Could you check a few things on this model? Use its own coordinates, in mm. Face numbers are marked on the shaded views. A direction names the side the tool comes from. Give positions to 0.01 mm unless a question says otherwise; leave off trailing zeros. Loops run counter-clockwise (first coordinate to the right, second up) from the corner with the lowest first, then second, coordinate; pieces in that order, holes last. Notation, with made-up numbers: (-5.5, 75.25) -> (35.5, 75.25) arc R27 cw to (35.5, 112.25) -> close; hole circle Ø5 at (68, -28). An arc over 180 degrees is marked (long way). Write each question's results on one line, items separated by ' | '. Start each with the question number.
Q1. If we section it at C-C, the plane y = -1: List the corners of the cut face in (x, z) for me, plus the area to 3 significant figures.
Q2. If we section it at D-D, the plane z = 0: List the corners of the cut face in (x, y) for me, plus the area to 3 significant figures.
Q3. We'd pull the mould along Z, two halves only. Please class the marked faces 5, 6, 7 and 8: released by +Z, released by -Z, zero draft, split by the parting line, or undercut.
Q4. If I drill on line 1 along X through (y, z) = (-1.3, 0); line 2 along Y through (x, z) = (4, 2.75); line 3 along Z through (x, y) = (-16, -1.7), over which ranges is the centre line in solid material (lowest first)?
Q5. Which directions (+Z, -Z, +X, -X, +Y, -Y) give clear straight access to the entire face, cutting with the end or side of a thin tool? Please do the marked faces 1, 2, 3 and 4.
Q6. If we section it at A-A, the plane z = 10.25: List the corners of the cut face in (x, y) for me, plus the area to 3 significant figures.
Q7. If we section it at B-B, the plane x = -12: List the corners of the cut face in (y, z) for me.
Q8. Will these pins go through, and if not, where does the flat tip stop? P1, Ø2.5, axis at x = 6, y = -6.5, coming from the -Z side; P2, Ø6, axis at y = -5.5, z = 5.5, coming from the +X side; P3, Ø6.5, axis at y = -10, z = 12.5, coming from the -X side.
from build123d import *

# Parameters (mm, degrees)
F0_R     = 3
F0_W     = 20
F0_H     = 8
F1_DEPTH = 14
F2_T     = -3
F3_DEPTH = 14


with BuildPart() as f1:
    # F0 (on Front) → F1 (new body)
    with BuildSketch(Plane.XZ):
        with BuildLine():
            Line((-4, 8), (-16, 8))
            ThreePointArc((-16, 8), (-24, 0), (-16, -8))
            Line((-16, -8), (16, -8))
            ThreePointArc((16, -8), (24, 0), (16, 8))
            Line((16, 8), (-4, 8))
        make_face()
        with Locations((-16, 0)):
            Circle(F0_R, mode=Mode.SUBTRACT)
        with Locations((16, 0)):
            Circle(F0_R, mode=Mode.SUBTRACT)
        with Locations((6, 12)):
            Rectangle(F0_W, F0_H)
        with Locations((-16, 0)):
            Circle(F0_R)
        with Locations((16, 0)):
            Circle(F0_R)
    extrude(amount=F1_DEPTH)

    # F2
    f2_openings = [f1.faces().sort_by_distance(p)[0] for p in [
        (-4, -7, 12),
        (-10, -7, 8),
        (-24, -7, 0),
        (0, -7, -8),
        (24, -7, 0),
        (16, -7, 12),
    ]]
    offset(amount=F2_T, openings=f2_openings)

    # F0 (on Front) → F3 (cut)
    with BuildSketch(Plane.XZ):
        with Locations((16, 0)):
            Circle(F0_R)
        with Locations((-16, 0)):
            Circle(F0_R)
    extrude(amount=F3_DEPTH, mode=Mode.SUBTRACT)


solid = f1.part
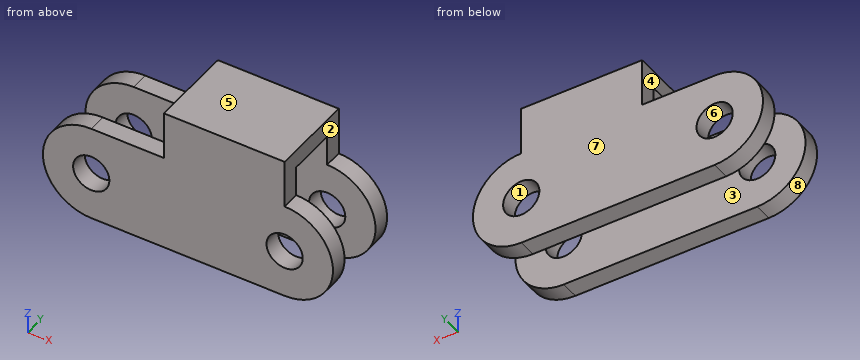
Final values:
1) outline: (-16, -8) -> (16, -8) arc R8 ccw to (16, 8) -> (16, 16) -> (-4, 16) -> (-4, 8) -> (-16, 8) arc R8 ccw to start; hole circle Ø6 at (-16, 0); hole circle Ø6 at (16, 0) | area: 817 mm²
2) outline: (-24, -14) -> (-19, -14) -> (-19, -11) -> (-24, -11) -> close; (-24, -3) -> (-19, -3) -> (-19, 0) -> (-24, 0) -> close; (-13, -14) -> (13, -14) -> (13, -11) -> (-13, -11) -> close; (-13, -3) -> (13, -3) -> (13, 0) -> (-13, 0) -> close; (19, -14) -> (24, -14) -> (24, -11) -> (19, -11) -> close; (19, -3) -> (24, -3) -> (24, 0) -> (19, 0) -> close | area: 216 mm²
3) face 5: released by +Z | face 6: undercut | face 7: zero draft | face 8: split by the parting line
4) line 1: x = -24 to -19, -13 to 13, 19 to 24 | line 2: y = -14 to -11, -3 to 0 | line 3: z = -8 to -3, 3 to 8
5) face 1: +Y, -Y | face 2: +Z, +X, +Y, -Y | face 3: -Z, +X, -X | face 4: +Z, -X, +Y, -Y
6) outline: (-4, -14) -> (16, -14) -> (16, -11) -> (-4, -11) -> close; (-4, -3) -> (16, -3) -> (16, 0) -> (-4, 0) -> close | area: 120 mm²
7) outline: (-14, -8) -> (-11, -8) -> (-11, 8) -> (-14, 8) -> close; (-3, -8) -> (0, -8) -> (0, 8) -> (-3, 8) -> close
8) P1: stops at z = 13 | P2: stops at x = 23.02 | P3: stops at x = -4
